from build123d import *

# Parameters (mm, degrees)
SKETCH3_W = 4
SKETCH3_H = 30


with BuildPart() as part:
    # Sweep1: sweep along a path in Sketch1
    with BuildLine(Plane(origin=(0, 0, 0), x_dir=(1, 0, 0), z_dir=(0, 1, 0))) as sweep1_path:
        Line((-0.05, 100.5), (0.05, 100.5))
        ThreePointArc((0.05, 100.5), (6.201828996, 97.951828996), (8.75, 91.8))
        Line((8.75, 91.8), (8.75, -91.8))
        ThreePointArc((8.75, -91.8), (6.201828996, -97.951828996), (0.05, -100.5))
        Line((0.05, -100.5), (-0.05, -100.5))
        ThreePointArc((-0.05, -100.5), (-6.201828996, -97.951828996), (-8.75, -91.8))
        Line((-8.75, -91.8), (-8.75, 91.8))
        ThreePointArc((-8.75, 91.8), (-6.201828996, 97.951828996), (-0.05, 100.5))
    # Sketch3 → Sweep1 (sweep)
    with BuildSketch(Plane.XY):
        with Locations((8.75, 0)):
            Rectangle(SKETCH3_W, SKETCH3_H)
    sweep(path=sweep1_path.line)


solid = part.part
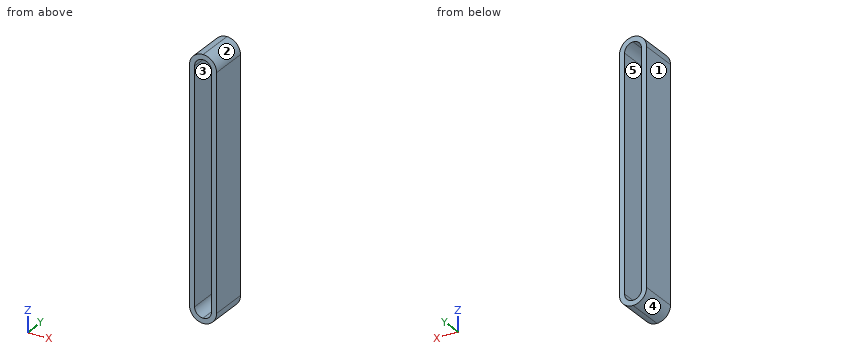
Here's how the part is built. I have some questions about the finished solid (model axes, mm). Face numbers are marked on the shaded views. A direction names the side the tool comes from. Coordinates: 2 decimals unless noted, no trailing zeros. Order: outer loops, then holes, each group sorted by start corner. A loop starts at its lowest first (then second) coordinate and runs counter-clockwise, first axis right, second up. Notation, with made-up numbers: M 84.25,39.25 L 93.25,39.25 A8 cw 93.25,43.25 Z; hole C 18,47 d1. An arc over 180 degrees is marked long. Answer as CSV lines item,"result".
Item 1: Imagine slicing it at B-B on y = 8.25. Write out the boundary of the cut face in (x, z).
Results found:
outline,"M -10.75,-91.8 A10.7 ccw -0.05,-102.5 L 0.05,-102.5 A10.7 ccw 10.75,-91.8 L 10.75,91.8 A10.7 ccw 0.05,102.5 L -0.05,102.5 A10.7 ccw -10.75,91.8 Z; hole M -6.75,-91.8 A6.7 ccw -0.05,-98.5 L 0.05,-98.5 A6.7 ccw 6.75,-91.8 L 6.75,91.8 A6.7 ccw 0.05,98.5 L -0.05,98.5 A6.7 ccw -6.75,91.8 Z"
Item 2: For pin 1 (4 mm diameter, centred on x = 2, y = -9.5, fed in from -Z); pin 2 (1.5 mm diameter, centred on x = 5.5, y = -11.5, fed in from +Z), each with a flat end and sliding along its axis, tell me the tip position at first contact or that it passes through.
Results found:
pin 1,"z = -102.5"
pin 2,"z = 101.41"
Item 3: If I drill on line 1 (X direction, y = 5.25, z = -1.5); line 2 (Z direction, x = -0.75, y = 4.25); line 3 (Z direction, x = 1.5, y = -5.5), over which ranges is the centre line in solid material (lowest first)?
Results found:
line 1,"-10.75 to -6.75, 6.75 to 10.75"
line 2,"-102.48 to -98.46, 98.46 to 102.48"
line 3,"-102.4 to -98.34, 98.34 to 102.4"
Item 4: Imagine slicing it at D-D on x = -8.5. Write out the boundary of the cut face in (y, z), plus the area to 3 significant figures.
Results found:
outline,"M -15,-98.36 L 15,-98.36 L 15,98.36 L -15,98.36 Z"
area,"5,900 mm2"
Item 5: On a 3-axis mill with a long thin cutter (end or side, diameter ignored), from which of +Z, -Z, +X, -X, +Y, -Y can I reach the whole of each face in a straight line? I mean the marked faces 4 and 5. Say none if no direction works.
Results found:
face 4,"-Z, -X, +Y, -Y"
face 5,"+Y, -Y"
Item 6: Imagine slicing it at C-C on x = 4.25. Write out the boundary of the cut face in (y, z), plus the area to 3 significant figures.
Results found:
outline,"M -15,-101.64 L 15,-101.64 L 15,-97.02 L -15,-97.02 Z; M -15,97.02 L 15,97.02 L 15,101.64 L -15,101.64 Z"
area,"277 mm2"
Item 7: Imagine slicing it at A-A on z = 68. Write out the boundary of the cut face in (x, y).
Results found:
outline,"M -10.75,-15 L -6.75,-15 L -6.75,15 L -10.75,15 Z; M 6.75,-15 L 10.75,-15 L 10.75,15 L 6.75,15 Z"
Item 8: We'd pull the mould along X, two halves only. Please class the marked faces 1, 2 and 3: +X half, -X half, draft (parallel to the pull), parting line (faces both ways), or undercut.
Results found:
face 1,"-X half"
face 2,"+X half"
face 3,"undercut"
